Geometry: final body of the model. Coordinates: model frame, mm. A direction names the side the tool comes from. Round coordinates to 2 decimals unless told otherwise and drop trailing zeros. Loops run counter-clockwise (first coordinate to the right, second up) from the corner with the lowest first, then second, coordinate; pieces in that order, holes last. Notation, with made-up numbers: (84.25, 2) -> (98.25, 2) arc R24 ccw to (98.25, 38) -> close; hole circle Ø6 at (-26, 12.5). An arc over 180 degrees is marked (long way). Answer in a Markdown table with one row per item.
```python
from build123d import *

# Parameters (mm, degrees)
F0_W     = 156.916313
F0_H     = 78.295462
F1_DEPTH = 25
F2_R     = 5
F3_DEPTH = 25


with BuildPart() as f1:
    # F0 (on Front) → F1 (new body)
    with BuildSketch(Plane.XZ):
        with Locations((78.458157, 39.147731)):
            Rectangle(F0_W, F0_H)
    extrude(amount=F1_DEPTH)

    # F2 (on face) → F3 (join)
    with BuildSketch(Plane.XZ.offset(25)):
        with Locations((24.000163, 41.481324)):
            Circle(F2_R)
        with Locations((79.000163, 41.481324)):
            Circle(F2_R)
        with Locations((124.000163, 41.481324)):
            Circle(F2_R)
    extrude(amount=F3_DEPTH)


solid = f1.part
```
Item 1: Line query: probe 1 along Y at (x, z) = (65, 59); probe 2 along Z at (x, y) = (79, -27); probe 3 along Z at (x, y) = (22, -41.5). Output: solid intervals per line, ascending. Write a range as [from, to].
Answer:
| item | result |
|---|---|
| probe 1 | y = [-25, 0] |
| probe 2 | z = [36.48, 46.48] |
| probe 3 | z = [36.9, 46.06] |
Item 2: Pin query (flat end, axial travel): pin 1 Ø8 at (x, z) = (88.5, 68.5) entering from -Y; pin 2 Ø8 at (y, z) = (-26.5, 55.5) entering from -X; pin 3 Ø2 at (y, z) = (-34.5, 46) entering from +X; pin 4 Ø6 at (y, z) = (-38, 37.5) entering from -X. Return the tip coordinate at first contact, or that it passes through.
Answer:
| item | result |
|---|---|
| pin 1 | stops at y = -25 |
| pin 2 | stops at x = 0 |
| pin 3 | stops at x = 127.55 |
| pin 4 | stops at x = 19.1 |
Item 3: Draft query along X for faces 3 (the face through (0, -12, 39)), 4 (the face through (128.77, -37.33, 42.98)), 5 (the face through (24, -50, 42)). Return one class per face: pulls with the +X half, pulls with the -X half, needs draft (parallel to the pull), parting line crosses it, or undercut.
Answer:
| item | result |
|---|---|
| face 3 | pulls with the -X half |
| face 4 | undercut |
| face 5 | needs draft |
Item 4: Cut plane C-C (x = 145). Output: boundary loops of the cut face in (y, z), then the cut area to 3 significant figures.
Answer:
| item | result |
|---|---|
| outline | (-25, 0) -> (0, 0) -> (0, 78.3) -> (-25, 78.3) -> close |
| area | 1,960 mm² |
Item 5: Cut plane B-B (z = 8.5). Output: boundary loops of the cut face in (x, y), then the cut area to 3 significant figures.
Answer:
| item | result |
|---|---|
| outline | (0, -25) -> (156.92, -25) -> (156.92, 0) -> (0, 0) -> close |
| area | 3,920 mm² |
Item 6: Cut plane A-A (y = -26.5). Output: boundary loops of the cut face in (x, z), then the cut area to 3 significant figures.
Answer:
| item | result |
|---|---|
| outline | circle Ø10 at (24, 41.48); circle Ø10 at (79, 41.48); circle Ø10 at (124, 41.48) |
| area | 236 mm² |
Item 7: Reachability of faces 1 (the face through (26.688, -37.325, 45.697)), 2 (the face through (77, -12, 0)) from +Z, -Z, +X, -X, +Y, -Y: full face, straight path, thin tool, end or side. Return the list, or none.
Answer:
| item | result |
|---|---|
| face 1 | -Y |
| face 2 | -Z, +X, -X, +Y, -Y |
